CAD build for the part. Positions are in the model's coordinates, mm. Face numbers are marked on the shaded views. Round coordinates to 2 decimals unless told otherwise and drop trailing zeros. Write each loop counter-clockwise with the first axis right and the second up, starting at its lowest first coordinate (ties: lowest second). Pieces come first, ordered by that corner, then holes. Notation, with made-up numbers: (80, 76) - (136, 76) arc R35 ccw to (136, 115) - close; hole circle Ø8 at (72.5, 69). An arc over 180 degrees is marked (long way). Use one line per item in the form item = value. Start each with the question number.
Item 1: Band-saw the part on D-D, the plane y = 30. List the corners of the cut face in (x, z), and give its area (3 significant figures).
Item 2: Pull direction X, two halves, no side cores. Call the marked faces 1, 2, 3 and 4: +X half, -X half, draft (parallel to the pull), parting line (faces both ways), or undercut.
Item 3: Drill centre lines: L1, parallel to Z at x = 33, y = 30; L2, parallel to Y at x = -34, z = 30; L3, parallel to X at y = 36.5, z = 52. Where is each one in solid material? Low to high.
Item 4: Pin check, flat tips, straight feed: pin 1 (6.5 mm diameter, centred on x = -8.84, z = 38.84, fed in from -Y); pin 2 (2.5 mm diameter, centred on y = 0, z = 4.5, fed in from +X). Stop position of each tip, or through.
Item 5: Band-saw the part on C-C, the plane z = 4.5. List the corners of the cut face in (x, y).
Item 6: Band-saw the part on A-A, the plane y = 38.5. List the corners of the cut face in (x, z).
Item 7: Band-saw the part on B-B, the plane z = 30. Give the number of separate pieces and of enclosed holes in the cut face, and give its area (3 significant figures).
from build123d import *

# Parameters (mm, degrees)
RESSALTO_EXTRUS_O1_DEPTH = 60
ESBO_O2_R                = 4
CORTE_EXTRUS_O1_DEPTH    = 65
ESBO_O3_R                = 2.5
CORTE_EXTRUS_O2_DEPTH    = 10
RESSALTO_EXTRUS_O2_DEPTH = 5
RESSALTO_EXTRUS_O3_DEPTH = 5
ESBO_O6_R                = 2
CORTE_EXTRUS_O3_DEPTH    = 10
ESBO_O7_W                = 70
ESBO_O7_H                = 70
ESBO_O7_R                = 2
ESBO_O7_R_2              = 4
RESSALTO_EXTRUS_O4_DEPTH = 2.5
ESBO_O8_W                = 70
ESBO_O8_H                = 70
ESBO_O8_R                = 4
RESSALTO_EXTRUS_O5_DEPTH = 2.5
ESBO_O9_W                = 70
ESBO_O9_H                = 68
CORTE_EXTRUS_O4_DEPTH    = 2.5
ESBO_O10_W               = 70
ESBO_O10_H               = 68
CORTE_EXTRUS_O5_DEPTH    = 2.5
ESBO_O11_R               = 2
CORTE_EXTRUS_O6_DEPTH    = 70


with BuildPart() as part:
    # Esboço1 → Ressalto-extrusão1 (new body)
    with BuildSketch(Plane.XY):
        Polygon((32, -15), (32, 55), (-32, 55), (-32, -15), (-30, -15), (-30, -13), (-30, 53), (30, 53), (30, -13), (30, -15), align=None)
    extrude(amount=RESSALTO_EXTRUS_O1_DEPTH)

    # Esboço2 → Corte-extrusão1 (cut, through all)
    with BuildSketch(Plane(origin=(32, 0, 0), x_dir=(0, 0, -1), z_dir=(1, 0, 0))):
        with Locations((-30, 15)):
            Circle(ESBO_O2_R)
    extrude(amount=-CORTE_EXTRUS_O1_DEPTH, mode=Mode.SUBTRACT)

    # Esboço3 → Corte-extrusão2 (cut)
    with BuildSketch(Plane.XZ.offset(-53)):
        with Locations((-8.838834765, 38.838834765)):
            Circle(ESBO_O3_R)
        with Locations((-8.838834765, 21.161165235)):
            Circle(ESBO_O3_R)
        with Locations((8.838834765, 21.161165235)):
            Circle(ESBO_O3_R)
        with Locations((8.838834765, 38.838834765)):
            Circle(ESBO_O3_R)
    extrude(amount=-CORTE_EXTRUS_O2_DEPTH, mode=Mode.SUBTRACT)

    # Esboço4 → Ressalto-extrusão2 (add)
    with BuildSketch(Plane.XY.offset(60)):
        Polygon((-32, 55), (-32, -15), (-30, -15), (-30, 53), (30, 53), (30, -15), (32, -15), (32, 55), align=None)
    extrude(amount=RESSALTO_EXTRUS_O2_DEPTH)

    # Esboço5 → Ressalto-extrusão3 (add)
    with BuildSketch(Plane(origin=(0, 0, 0), x_dir=(-1, 0, 0), z_dir=(0, 0, -1))):
        Polygon((32, -15), (32, 55), (-32, 55), (-32, -15), (-30, -15), (-30, 53), (30, 53), (30, -15), align=None)
    extrude(amount=RESSALTO_EXTRUS_O3_DEPTH)

    # Esboço6 → Corte-extrusão3 (cut)
    with BuildSketch(Plane(origin=(32, 0, 0), x_dir=(0, 0, -1), z_dir=(1, 0, 0))):
        with Locations((-4.5, 0)):
            Circle(ESBO_O6_R)
        with Locations((-4.5, 30)):
            Circle(ESBO_O6_R)
        with Locations((-55.5, 0)):
            Circle(ESBO_O6_R)
        with Locations((-55.5, 30)):
            Circle(ESBO_O6_R)
    extrude(amount=-CORTE_EXTRUS_O3_DEPTH, mode=Mode.SUBTRACT)

    # Esboço7 → Ressalto-extrusão4 (add)
    with BuildSketch(Plane(origin=(32, 0, 0), x_dir=(0, 0, -1), z_dir=(1, 0, 0))):
        with Locations((-30, 20)):
            Rectangle(ESBO_O7_W, ESBO_O7_H)
        with Locations((-55.5, 0)):
            Circle(ESBO_O7_R, mode=Mode.SUBTRACT)
        with Locations((-55.5, 30)):
            Circle(ESBO_O7_R, mode=Mode.SUBTRACT)
        with Locations((-30, 15)):
            Circle(ESBO_O7_R_2, mode=Mode.SUBTRACT)
        with Locations((-4.5, 0)):
            Circle(ESBO_O7_R, mode=Mode.SUBTRACT)
        with Locations((-4.5, 30)):
            Circle(ESBO_O7_R, mode=Mode.SUBTRACT)
    extrude(amount=RESSALTO_EXTRUS_O4_DEPTH)

    # Esboço8 → Ressalto-extrusão5 (add)
    with BuildSketch(Plane.ZY.offset(32)):
        with Locations((30, 20)):
            Rectangle(ESBO_O8_W, ESBO_O8_H)
        with Locations((30, 15)):
            Circle(ESBO_O8_R, mode=Mode.SUBTRACT)
    extrude(amount=RESSALTO_EXTRUS_O5_DEPTH)

    # Esboço9 → Corte-extrusão4 (cut)
    with BuildSketch(Plane.ZY.offset(-30)):
        with Locations((30, 19)):
            Rectangle(ESBO_O9_W, ESBO_O9_H)
    extrude(amount=-CORTE_EXTRUS_O4_DEPTH, mode=Mode.SUBTRACT)

    # Esboço10 → Corte-extrusão5 (cut)
    with BuildSketch(Plane(origin=(-30, 0, 0), x_dir=(0, 0, -1), z_dir=(1, 0, 0))):
        with Locations((-30, 19)):
            Rectangle(ESBO_O10_W, ESBO_O10_H)
    extrude(amount=-CORTE_EXTRUS_O5_DEPTH, mode=Mode.SUBTRACT)

    # Esboço11 → Corte-extrusão6 (cut, through all)
    with BuildSketch(Plane(origin=(34.5, 0, 0), x_dir=(0, 0, -1), z_dir=(1, 0, 0))):
        with Locations((-30, -3.25)):
            Circle(ESBO_O11_R)
        with Locations((-30, 33.25)):
            Circle(ESBO_O11_R)
    extrude(amount=-CORTE_EXTRUS_O6_DEPTH, mode=Mode.SUBTRACT)


solid = part.part
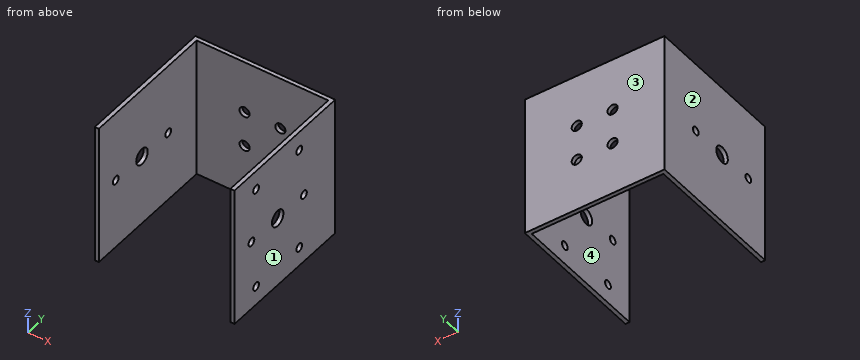
Determined:
q1.outline = (-34.5, -5) - (-32.5, -5) - (-32.5, 65) - (-34.5, 65) - close; (32.5, -5) - (34.5, -5) - (34.5, 2.5) - (32.5, 2.5) - close; (32.5, 6.5) - (34.5, 6.5) - (34.5, 53.5) - (32.5, 53.5) - close; (32.5, 57.5) - (34.5, 57.5) - (34.5, 65) - (32.5, 65) - close
q1.area = 264 mm²
q2.face_1 = +X half
q2.face_2 = -X half
q2.face_3 = draft
q2.face_4 = undercut
q3.L1 = -5 to 2.5, 6.5 to 53.5, 57.5 to 65
q3.L2 = -15 to -5.25, -1.25 to 11, 19 to 31.25, 35.25 to 55
q3.L3 = -34.5 to -32.5, 32.5 to 34.5
q4.pin_1 = 53
q4.pin_2 = -32.5
q5.outline = (-34.5, -15) - (-32.5, -15) - (-32.5, 53) - (32.5, 53) - (32.5, 32) - (34.5, 32) - (34.5, 55) - (-34.5, 55) - close; (32.5, -15) - (34.5, -15) - (34.5, -2) - (32.5, -2) - close; (32.5, 2) - (34.5, 2) - (34.5, 28) - (32.5, 28) - close
q6.outline = (-34.5, -5) - (-32.5, -5) - (-32.5, 65) - (-34.5, 65) - close; (32.5, -5) - (34.5, -5) - (34.5, 65) - (32.5, 65) - close
q7.separate_pieces = 7
q7.enclosed_holes = 0
q7.area = 346 mm²
